Verification items for the finished model (mm, model axes). A direction names the side the tool comes from. Coordinates: 2 decimals unless noted, no trailing zeros. Loops run counter-clockwise (first coordinate to the right, second up) from the corner with the lowest first, then second, coordinate; pieces in that order, holes last.
Q1. Material ranges on probe 1 along Y at (x, z) = (-4.5, -36); probe 2 along Z at (x, y) = (0, 944); probe 3 along Y at (x, z) = (-48.5, -7), recorded low to high.
Q2. Sectioned sample at C-C (y = 214.5). Enter the section's corners in (x, z).
Q3. Go/stop test with flat-tipped pins: P1, Ø4, axis at x = 135.5, z = 36.5, coming from the -Y side; P2, Ø17.5, axis at x = 18, y = 391.5, coming from the -Z side; P3, Ø8, axis at y = 998, z = 60, coming from the +X side. Record where each tip stops, or that it passes through.
Q4. Access from +Z, -Z, +X, -X, +Y, -Y to the whole of each face (thin tool, end or side, straight path). Record for faces 4 (the face through (-17, 1026, -55)), 5 (the face through (163.8, 1335.4, 65.1)), 6 (the face through (193.497, 1470.713, -65.14)).
Q5. Mould release check, pull along Y, two halves, no side actions. Record for faces 1 (the face through (188.97, 419.01, -65.14)), 2 (the face through (-73, 1009, 75)), 3 (the face through (202.966, 1628.233, 65.14)): +Y half, -Y half, draft (parallel to the pull), parting line (faces both ways), or undercut.
Q6. Sectioned sample at B-B (y = 1360.5). Enter the section's corners in (x, z), then the cut area to 3 significant figures.
Q7. Sectioned sample at A-A (z = 0). Enter the section's corners in (x, y).
```python
from build123d import *

# Parameters (mm, degrees)
SKETCH2_R           = 75
BOSS_EXTRUDE1_DEPTH = 1500
SHELL4_T            = 10
BOSS_EXTRUDE2_START = 75
SKETCH3_R           = 30
BOSS_EXTRUDE2_DEPTH = 20
SKETCH10_R          = 30
BOSS_EXTRUDE3_DEPTH = 95
SKETCH12_R          = 20
BOSS_EXTRUDE4_DEPTH = 75


with BuildPart() as part:
    # Sketch2 → Boss-Extrude1 (new body)
    with BuildSketch(Plane(origin=(0, 0, 0), x_dir=(1, 0, 0), z_dir=(0, 1, 0))):
        Circle(SKETCH2_R)
    extrude(amount=BOSS_EXTRUDE1_DEPTH)

    # Shell4 (no face opened: a closed hollow body)
    add(offset(amount=-SHELL4_T, mode=Mode.PRIVATE), mode=Mode.SUBTRACT)

    # Sketch3 → Boss-Extrude2 (add)
    with BuildSketch(Plane.XY.offset(BOSS_EXTRUDE2_START)):
        with BuildLine():
            Line((0, 450), (150, 450))
            ThreePointArc((150, 450), (189.137774485, 418.260424226), (166.164731025, 373.41173042))
            Line((166.164731025, 373.41173042), (0, 300))
            Line((0, 300), (0, 450))
        make_face()
        with BuildLine():
            Line((0, 1100), (0, 950))
            Line((0, 950), (-150, 950))
            ThreePointArc((-150, 950), (-189.137774485, 981.739575774), (-166.164731025, 1026.58826958))
            Line((-166.164731025, 1026.58826958), (0, 1100))
        make_face()
        with BuildLine():
            Line((0, 1200), (0, 1500))
            Line((0, 1500), (41.102417852, 1711.448791074))
            ThreePointArc((41.102417852, 1711.448791074), (91.875322735, 1759.447368481), (153.66563146, 1726.83281573))
            Line((153.66563146, 1726.83281573), (253.66563146, 1526.83281573))
            ThreePointArc((253.66563146, 1526.83281573), (259.897670219, 1496.497272164), (250.172245693, 1467.094897628))
            Line((250.172245693, 1467.094897628), (75, 1200))
            Line((75, 1200), (0, 1200))
        make_face()
        with Locations((200, 1500)):
            Circle(SKETCH3_R, mode=Mode.SUBTRACT)
    boss_extrude2 = extrude(amount=-BOSS_EXTRUDE2_DEPTH)

    # Mirror11: Boss-Extrude2 across plane
    add(boss_extrude2.mirror(Plane(origin=(0, 0, 0), x_dir=(1, 0, 0), z_dir=(0, 0, -1))))

    # Sketch10 → Boss-Extrude3 (add, symmetric)
    with BuildSketch(Plane.XY):
        with Locations((0, 60)):
            Circle(SKETCH10_R)
    extrude(amount=BOSS_EXTRUDE3_DEPTH, both=True)

    # Sketch12 → Boss-Extrude4 (add, symmetric)
    with BuildSketch(Plane.XY):
        with Locations((150, 410)):
            Circle(SKETCH12_R)
        with Locations((100, 1700)):
            Circle(SKETCH12_R)
        with Locations((-150, 990)):
            Circle(SKETCH12_R)
    extrude(amount=BOSS_EXTRUDE4_DEPTH, both=True)


solid = part.part
```
Geometry check:
1. probe 1: y = 0 to 10, 30.34 to 89.66, 1490 to 1500
1. probe 2: z = -75 to -65, 65 to 75
1. probe 3: y = 0 to 10, 1490 to 1500
2. outline: circle Ø150 at (0, 0); hole circle Ø130 at (0, 0)
3. P1: stops at y = 394.39
3. P2: stops at z = -75
3. P3: stops at x = 49.89
4. face 4: none
4. face 5: +Z, -Z, +X
4. face 6: +Z, -Z
5. face 1: undercut
5. face 2: draft
5. face 3: +Y half
6. outline: (0, -75) - (180.26, -75) - (180.26, -55) - (50.99, -55) arc R75 ccw to (50.99, 55) - (180.26, 55) - (180.26, 75) - (0, 75) arc R75 ccw to start; hole (0, -65) - (0, -55) - (34.64, -55) arc R65 ccw to (34.64, 55) - (0, 55) - (0, 65) arc R65 ccw to start
6. area: 10,700 mm2
7. outline: circle Ø40 at (-150, 990); (-75, 0) - (75, 0) - (75, 1500) - (-75, 1500) - close; circle Ø60 at (0, 60); circle Ø40 at (100, 1700); circle Ø40 at (150, 410); hole (-65, 10) - (65, 10) - (65, 1490) - (-65, 1490) - close
